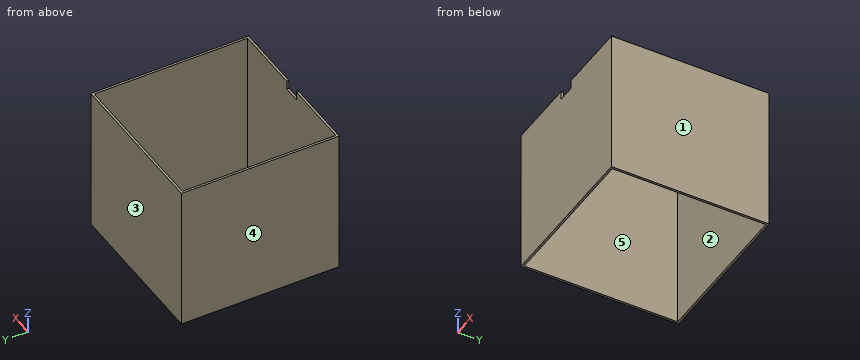
from build123d import *

# Parameters (mm, degrees)
F0_W     = 73.3
F0_H     = 73.3
F0_W_2   = 71.3
F0_H_2   = 71.3
F1_DEPTH = 68
F3_DEPTH = 5


with BuildPart() as f1:
    # F0 (on Top) → F1 (new body)
    with BuildSketch(Plane.XY):
        with Locations((36.65, -36.65)):
            Rectangle(F0_W, F0_H)
        with Locations((36.65, -36.65)):
            Rectangle(F0_W_2, F0_H_2, mode=Mode.SUBTRACT)
    extrude(amount=F1_DEPTH)

    # F2 (on face) → F3 (cut)
    with BuildSketch(Plane.XZ.offset(73.3)):
        Polygon((32.65, 64), (36.65, 64), (40.65, 64), (40.65, 68), (32.65, 68), align=None)
    extrude(amount=-F3_DEPTH, mode=Mode.SUBTRACT)


solid = f1.part
Build history of the part. All positions in model axes, mm. Face numbers are marked on the shaded views. A direction names the side the tool comes from. Give positions to 0.01 mm unless a question says otherwise; leave off trailing zeros. Order: outer loops, then holes, each group sorted by start corner. A loop starts at its lowest first (then second) coordinate and runs counter-clockwise, first axis right, second up. Notation, with made-up numbers: M -21,50 L -13,50 A21 cw -13,58 Z; hole C 80,-14.75 d4. An arc over 180 degrees is marked long. Use one line per item in the form item = value.
Q1. Pin check, flat tip, straight feed: P1, Ø10, axis at x = 62.5, y = -22.5, coming from the -Z side. Stop position of the tip, or through.
Conclusion:
P1 = through
Q2. Slice it at A-A, the plane x = 67. Write the cut outline in (y, z).
Conclusion:
outline = M -73.3,0 L -72.3,0 L -72.3,68 L -73.3,68 Z; M -1,0 L 0,0 L 0,68 L -1,68 Z
Q3. Slice it at C-C, the plane z = 57.5. Write the cut outline in (x, y), and give its area (3 significant figures).
Conclusion:
outline = M 0,-73.3 L 73.3,-73.3 L 73.3,0 L 0,0 Z; hole M 1,-72.3 L 72.3,-72.3 L 72.3,-1 L 1,-1 Z
area = 289 mm2
Q4. Which spindle directions (+Z, -Z, +X, -X, +Y, -Y) get a long thin tool onto all of the face, cutting with end or side? Do the marked faces 4 and 5. Say none if no direction does.
Conclusion:
face_4 = +Z, -Z, -X, +Y, -Y
face_5 = +Z, -Z
Q5. Wall check: probe 1 along X at (y, z) = (-10, 23); probe 2 along Y at (x, z) = (12, 54). Give the ranges that are in metal, low to high.
Conclusion:
probe_1 = 0 to 1, 72.3 to 73.3
probe_2 = -73.3 to -72.3, -1 to 0
Q6. Slice it at B-B, the plane y = -57.5. Write the cut outline in (x, z).
Conclusion:
outline = M 0,0 L 1,0 L 1,68 L 0,68 Z; M 72.3,0 L 73.3,0 L 73.3,68 L 72.3,68 Z
Q7. Pull direction Y, two halves, no side cores. Call the marked faces 1, 2 and 3: released by +Y, released by -Y, zero draft, split by the parting line, or undercut.
Conclusion:
face_1 = zero draft
face_2 = undercut
face_3 = released by +Y
